Here's how the part is built. I have some questions about the finished solid (model axes, mm). Face numbers are marked on the shaded views. A direction names the side the tool comes from. Round coordinates to 2 decimals unless told otherwise and drop trailing zeros. Write each loop counter-clockwise with the first axis right and the second up, starting at its lowest first coordinate (ties: lowest second). Pieces come first, ordered by that corner, then holes. Notation, with made-up numbers: M 57,80 L 74,80 A26 cw 74,95 Z; hole C 68,30 d4. An arc over 180 degrees is marked long. Use one line per item in the form item = value. Start each with the question number.
Q1. I need wall thicknesses on line 1 along Z through (x, y) = (3, -12); line 2 along X through (y, z) = (31.5, -2); line 3 along Y through (x, z) = (8.5, -29.5). Which ranges of each line are inside material? Lowest first, please. Write a range as from..to.
Q2. I want a section at B-B on x = -9. List the corners of the cut face in (y, z) for me.
Q3. For the marked faces 1, 2, 3 and 4, which set-ups out of +Z, -Z, +X, -X, +Y, -Y let a thin tool reach every point of the face, with its end or its side?
Q4. I want a section at C-C on z = -3. List the corners of the cut face in (x, y) for me, and give its area (3 significant figures).
Q5. I'm going to push flat-ended pins straight in: pin 1 Ø1.9 at (x, z) = (3, -8) entering from -Y; pin 2 Ø25 at (y, z) = (16, -10) entering from +X; pin 3 Ø4.5 at (x, y) = (-7.5, 22.5) entering from -Z; pin 4 Ø1.5 at (x, z) = (0.5, -15) entering from +Y. Where does each tip first touch, or does it pass through?
Q6. I want a section at A-A on y = 24. List the corners of the cut face in (x, z) for me, and give its area (3 significant figures).
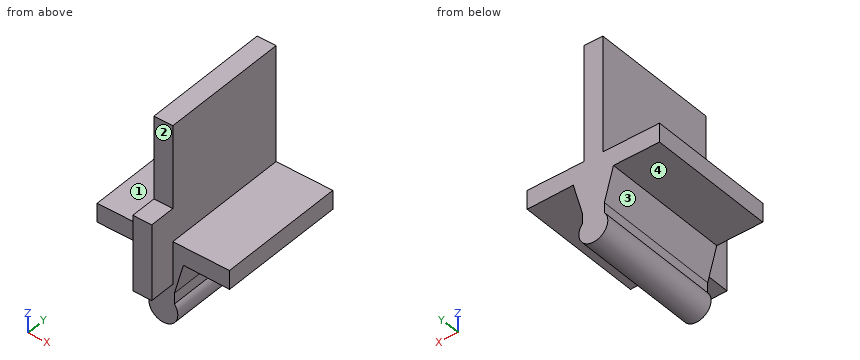
```python
from build123d import *

# Parameters (mm, degrees)
BOSS_EXTRUDE1_DEPTH = 27
BOSS_EXTRUDE2_DEPTH = 5.5
SCALE4_SCALE        = 1.55


with BuildPart() as part:
    # Sketch1 → Boss-Extrude1 (new body)
    with BuildSketch(Plane(origin=(0, 0, 0), x_dir=(1, 0, 0), z_dir=(0, 1, 0))):
        with BuildLine():
            Line((5.744481064, 28.356552325), (5.744481064, 3.856552325))
            Line((5.744481064, 3.856552325), (1.744481064, 3.856552325))
            Line((1.744481064, 3.856552325), (1.744481064, 28.356552325))
            Line((1.744481064, 28.356552325), (-10.255518936, 28.356552325))
            Line((-10.255518936, 28.356552325), (-10.255518936, 32.356552325))
            Line((-10.255518936, 32.356552325), (-0.505518936, 32.356552325))
            Line((-0.505518936, 32.356552325), (1.40938179, 39.233461433))
            Line((1.40938179, 39.233461433), (1.40938179, 41.356552325))
            ThreePointArc((1.40938179, 41.356552325), (3.744481064, 46.398404602), (6.079580338, 41.356552325))
            Line((6.079580338, 41.356552325), (6.079580338, 39.078120853))
            Line((6.079580338, 39.078120853), (7.994481064, 32.202963761))
            Line((7.994481064, 32.202963761), (17.744481064, 32.356552325))
            Line((17.744481064, 32.356552325), (17.744481064, 28.356552325))
            Line((17.744481064, 28.356552325), (5.744481064, 28.356552325))
        make_face()
    extrude(amount=BOSS_EXTRUDE1_DEPTH)

    # Sketch2 → Boss-Extrude2 (add)
    with BuildSketch(Plane.XZ):
        Polygon((1.744481064, -21.356552325), (5.744481064, -21.356552325), (5.744481064, -28.356552325), (5.744481064, -37.356552325), (1.744481064, -37.356552325), (1.744481064, -28.356552325), align=None)
    extrude(amount=BOSS_EXTRUDE2_DEPTH)


with BuildPart() as part_1:
    # Scale4: scaled about (3.722745038, 12.801128323, -27.923162877)
    add(part.part.scale(SCALE4_SCALE).moved(Location((-2.047509771, -7.040620578, 15.357739582))))


solid = part_1.part
```
Reported:
q1.line_1 = -42.54..-17.74
q1.line_2 = 0.66..6.86
q1.line_3 = -7.04..34.81
q2.outline = M -7.04,-34.79 L 34.81,-34.79 L 34.81,-28.59 L -7.04,-28.59 Z
q3.face_1 = +Z, -X, +Y, -Y
q3.face_2 = +Z, +X, -X, -Y
q3.face_3 = -X, +Y, -Y
q3.face_4 = -Z, -X, +Y, -Y
q4.outline = M 0.66,-7.04 L 6.86,-7.04 L 6.86,34.81 L 0.66,34.81 Z
q4.area = 259 mm^2
q5.pin_1 = -7.04
q5.pin_2 = 6.86
q5.pin_3 = -34.79
q5.pin_4 = 34.81
q6.outline = M -17.94,-34.79 L -2.83,-34.79 L 0.14,-45.45 L 0.14,-48.74 A4.75 ccw long 7.38,-48.74 L 7.38,-45.21 L 10.34,-34.56 L 25.46,-34.79 L 25.46,-28.59 L 6.86,-28.59 L 6.86,9.38 L 0.66,9.38 L 0.66,-28.59 L -17.94,-28.59 Z
q6.area = 697 mm^2
